Check sheet for the modelled part. Datum: model origin and axes. Units: mm. A direction names the side the tool comes from. Give positions to 0.01 mm unless a question says otherwise; leave off trailing zeros. Order: outer loops, then holes, each group sorted by start corner. A loop starts at its lowest first (then second) coordinate and runs counter-clockwise, first axis right, second up. Notation, with made-up numbers: (-26.5, -29.5) - (12.5, -29.5) arc R24 cw to (12.5, -18.5) - close; hole circle Ø5 at (-32, -19.75). An arc over 180 degrees is marked (long way). Answer in a Markdown table with one row per item.
from build123d import *

# Parameters (mm, degrees)
EXTRUDE_1_DEPTH     = 15
EXTRUDE_2_DEPTH     = 20
CUT_EXTRUDE_1_DEPTH = 20


with BuildPart() as part:
    # 草圖1 → 填料-伸長1 (new body)
    with BuildSketch(Plane.XY):
        Polygon((0, 0), (20, 0), (15, 5), (10, 5), (10, 20), (0, 20), align=None)
    extrude_1 = extrude(amount=EXTRUDE_1_DEPTH)

    # 草圖2 → 填料-伸長2 (add)
    with BuildSketch(Plane.XY):
        with BuildLine():
            ThreePointArc((0, 10), (7.071067812, 12.928932188), (10, 20))
            Line((10, 20), (5, 20))
            ThreePointArc((5, 20), (3.535533906, 16.464466094), (0, 15))
            Line((0, 15), (0, 10))
        make_face()
    extrude_2 = extrude(amount=EXTRUDE_2_DEPTH)

    # 草圖2<3> → 除料-伸長1 (cut)
    with BuildSketch(Plane.XY):
        with BuildLine():
            ThreePointArc((0, 15), (3.535533906, 16.464466094), (5, 20))
            Line((5, 20), (0, 20))
            Line((0, 20), (0, 15))
        make_face()
    cut_extrude_1 = extrude(amount=CUT_EXTRUDE_1_DEPTH, mode=Mode.SUBTRACT)

    # 鏡射1: 填料-伸長1, 填料-伸長2, 除料-伸長1 across plane
    add(extrude_1.mirror(Plane(origin=(0, 0, 0), x_dir=(0, 0, 1), z_dir=(1, 0, 0))))
    add(extrude_2.mirror(Plane(origin=(0, 0, 0), x_dir=(0, 0, 1), z_dir=(1, 0, 0))))
    add(cut_extrude_1.mirror(Plane(origin=(0, 0, 0), x_dir=(0, 0, 1), z_dir=(1, 0, 0))), mode=Mode.SUBTRACT)


solid = part.part
(1) Cross-section at C-C, the plane x = -6. Record the cut outline in (y, z).
Geometry says:
| item | result |
|---|---|
| outline | (0, 0) - (20, 0) - (20, 20) - (12, 20) - (12, 15) - (0, 15) - close |
(2) Access from +Z, -Z, +X, -X, +Y, -Y to the whole of each face (thin tool, end or side, straight path). Record for faces 1 (the flat face through (-13, 5, 7)), 2 (the flat face through (13, 5, 7)), 3 (the flat face through (-8, 20, 10)).
Geometry says:
| item | result |
|---|---|
| face 1 | +Z, -Z, -X, +Y |
| face 2 | +Z, -Z, +X, +Y |
| face 3 | +Z, -Z, +X, -X, +Y |
(3) Cross-section at D-D, the plane y = 9.25. Record the cut outline in (x, z).
Geometry says:
| item | result |
|---|---|
| outline | (-10, 0) - (10, 0) - (10, 15) - (-10, 15) - close |
(4) Thickness scan on L1, parallel to X at y = 12.5, z = 2; L2, parallel to Y at x = 14, z = 1.5; L3, parallel to Z at x = 4.5, y = 2. Record the ranges inside material, lowest first.
Geometry says:
| item | result |
|---|---|
| L1 | -10 to 10 |
| L2 | 0 to 5 |
| L3 | 0 to 15 |
(5) Gauge pin test, flat ends, axial feed: P1, Ø10, axis at x = 8.5, y = 11.5, coming from the +Z side; P2, Ø12, axis at x = -15.5, y = 11.5, coming from the +Z side; P3, Ø2, axis at y = 4.5, z = 8, coming from the +X side; P4, Ø7.5, axis at y = 14.5, z = 9, coming from the -X side. Record the tip position at first contact, or that the pin passes through.
Geometry says:
| item | result |
|---|---|
| P1 | z = 20 |
| P2 | z = 15 |
| P3 | x = 16.5 |
| P4 | x = -10 |
(6) Cross-section at A-A, the plane z = 12. Record the cut outline in (x, y).
Geometry says:
| item | result |
|---|---|
| outline | (-20, 0) - (20, 0) - (15, 5) - (10, 5) - (10, 20) - (5, 20) arc R5 cw to (-5, 20) - (-10, 20) - (-10, 5) - (-15, 5) - close |
(7) Cross-section at B-B, the plane y = 17.5. Record the cut outline in (x, z).
Geometry says:
| item | result |
|---|---|
| outline | (-10, 0) - (-4.33, 0) - (-4.33, 20) - (-9.68, 20) - (-9.68, 15) - (-10, 15) - close; (4.33, 0) - (10, 0) - (10, 15) - (9.68, 15) - (9.68, 20) - (4.33, 20) - close |
